Source: CAD feature listing. Evaluate the final solid. Frame: model axes, mm. Coordinates: 2 decimals unless noted, no trailing zeros. Loops run counter-clockwise (first coordinate to the right, second up) from the corner with the lowest first, then second, coordinate; pieces in that order, holes last. Notation, with made-up numbers: (34, -3) - (72, -3) arc R29 ccw to (72, 26) - close; hole circle Ø1 at (84, 9). An arc over 180 degrees is marked (long way). Write item = value, one per line. Start each with the question number.
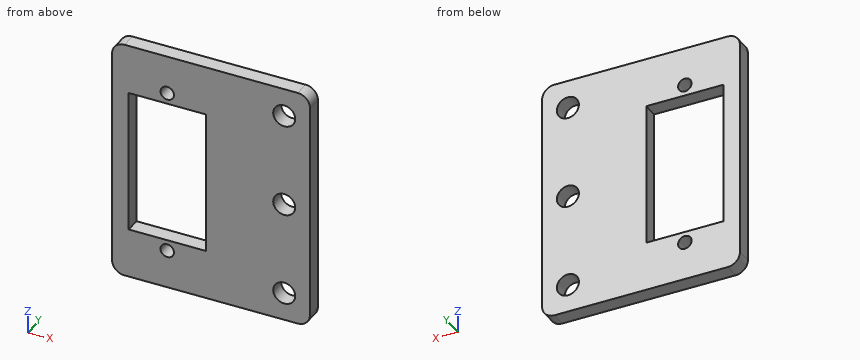
from build123d import *

# Parameters (mm, degrees)
SKETCH1_W             = 32.299999994
SKETCH1_H             = 39.7
PLATE_SIZE_DEPTH      = 2.5
SKETCH2_W             = 12.6
SKETCH2_H             = 23.5
SERVO_CLEARANCE_DEPTH = 3.5
M2_CLEARANCE_HOLE1_D  = 2.2
M3_CLEARANCE_HOLE1_D  = 3.6
CORNER_FILLET1_R      = 2


with BuildPart() as part:
    # Sketch1 → Plate Size (new body)
    with BuildSketch(Plane(origin=(0, 0, 0), x_dir=(1, 0, 0), z_dir=(0, 1, 0))):
        with Locations((7.149999997, 0)):
            Rectangle(SKETCH1_W, SKETCH1_H)
    extrude(amount=-PLATE_SIZE_DEPTH)

    # Sketch2 → Servo Clearance (cut, through all)
    with BuildSketch(Plane(origin=(0, 0, 0), x_dir=(1, 0, 0), z_dir=(0, 1, 0))):
        Rectangle(SKETCH2_W, SKETCH2_H)
    extrude(amount=-SERVO_CLEARANCE_DEPTH, mode=Mode.SUBTRACT)

    # M2 Clearance Hole1 (through all)
    with Locations(Plane(origin=(0, 0, 0), x_dir=(1, 0, 0), z_dir=(0, 1, 0))):
        with Locations((0, -13.55), (0, 13.55)):
            Hole(M2_CLEARANCE_HOLE1_D / 2)

    # M3 Clearance Hole1 (through all)
    with Locations(Plane(origin=(0, 0, 0), x_dir=(1, 0, 0), z_dir=(0, 1, 0))):
        with Locations((19.099999994, -15.25), (19.099999994, 0), (19.099999994, 15.25)):
            Hole(M3_CLEARANCE_HOLE1_D / 2)

    # Corner Fillet1
    corner_fillet1_edges = [part.edges().sort_by_distance(p)[0] for p in [
        (-9, -1.25, -19.85),
        (23.299999994, -1.25, -19.85),
        (23.299999994, -1.25, 19.85),
        (-9, -1.25, 19.85),
    ]]
    fillet(corner_fillet1_edges, radius=CORNER_FILLET1_R)


solid = part.part
Item 1: Cut plane C-C (x = 0). Return the cut outline in (y, z), then the cut area to 3 significant figures.
Item 2: Cut plane A-A (z = -11). Return the cut outline in (x, y).
Item 3: Material intervals for L1, parallel to Z at x = 19.1, y = -1.05; L2, parallel to Z at x = 18.5, y = -1; L3, parallel to X at y = -1.6, z = 15.25, sorted ascending. Write a range as [from, to].
Item 4: Cut plane B-B (y = -0.8). Return the cut outline in (x, z).
Item 5: Cut plane D-D (x = -3.5). Return the cut outline in (y, z).
Responses:
q1.outline = (-2.5, -19.85) - (0, -19.85) - (0, -14.65) - (-2.5, -14.65) - close; (-2.5, -12.45) - (0, -12.45) - (0, -11.75) - (-2.5, -11.75) - close; (-2.5, 11.75) - (0, 11.75) - (0, 12.45) - (-2.5, 12.45) - close; (-2.5, 14.65) - (0, 14.65) - (0, 19.85) - (-2.5, 19.85) - close
q1.area = 29.5 mm2
q2.outline = (-9, -2.5) - (-6.3, -2.5) - (-6.3, 0) - (-9, 0) - close; (6.3, -2.5) - (23.3, -2.5) - (23.3, 0) - (6.3, 0) - close
q3.L1 = [-19.85, -17.05], [-13.45, -1.8], [1.8, 13.45], [17.05, 19.85]
q3.L2 = [-19.85, -16.95], [-13.55, -1.7], [1.7, 13.55], [16.95, 19.85]
q3.L3 = [-9, 17.3], [20.9, 23.3]
q4.outline = (-9, -17.85) arc R2 ccw to (-7, -19.85) - (21.3, -19.85) arc R2 ccw to (23.3, -17.85) - (23.3, 17.85) arc R2 ccw to (21.3, 19.85) - (-7, 19.85) arc R2 ccw to (-9, 17.85) - close; hole (-6.3, -11.75) - (6.3, -11.75) - (6.3, 11.75) - (-6.3, 11.75) - close; hole circle Ø2.2 at (0, -13.55); hole circle Ø2.2 at (0, 13.55); hole circle Ø3.6 at (19.1, -15.25); hole circle Ø3.6 at (19.1, 0); hole circle Ø3.6 at (19.1, 15.25)
q5.outline = (-2.5, -19.85) - (0, -19.85) - (0, -11.75) - (-2.5, -11.75) - close; (-2.5, 11.75) - (0, 11.75) - (0, 19.85) - (-2.5, 19.85) - close
